The listing builds one solid part. Answer for the finished solid, in the listing's coordinates (mm). A direction names the side the tool comes from. Give positions to 0.01 mm unless a question says otherwise; leave off trailing zeros. Loops run counter-clockwise (first coordinate to the right, second up) from the corner with the lowest first, then second, coordinate; pieces in that order, holes last. Notation, with made-up numbers: M 9,74 L 25,74 A18 ccw 25,101 Z; hole C 73,78 d2. An arc over 180 degrees is marked long. Use one line per item in the form item = value. Start each with the question number.
1. The part is cut by section C-C (z = 10.75). Write down the section's boundary in (x, y), and give its area (3 significant figures).
2. The part is cut by section D-D (x = 7.25). Write down the section's boundary in (y, z), and give its area (3 significant figures).
3. Each of these flat-tipped pins is pushed along its axis until it touches: pin 1 Ø3 at (x, y) = (0, 12) entering from -Z; pin 2 Ø3 at (y, z) = (4, 0) entering from +X; pin 3 Ø2.5 at (y, z) = (14, 6.5) entering from +X. Where does it stop, or does it pass through?
4. Straight lines are drawn through the part: line 1 (Y direction, x = -3.75, z = 10); line 2 (Y direction, x = -4, z = 1); line 3 (Z direction, x = -5.25, y = 3). For each, find the intervals that lie inside material, in ascending order. Write a range as from..to.
5. The mould has two halves that part along Y. Classify faces 1 (the face through (5, 2.4, 4)), 2 (the face through (-3, 13, 9)), 3 (the face through (8, 9, 6)): released by +Y, released by -Y, zero draft, split by the parting line, or undercut.
6. The part is cut by section B-B (z = 0.5). Write down the section's boundary in (x, y).
7. The part is cut by section A-A (x = -5.5). Write down the section's boundary in (y, z).
8. For faces 4 (the face through (5, 5.75, 10)), 5 (the face through (-7.5, 12, 6)), 6 (the face through (-0.208, 13.586, 2.028)), 7 (the face through (-5, 2.4, 4)), 8 (the face through (0, 9, 9)), determine the directions among +Z, -Z, +X, -X, +Y, -Y from which every point of the face is accessible in a straight line to the end or side of a thin tool.
from build123d import *

# Parameters (mm, degrees)
BOSS_EXTRUDE1_DEPTH = 13
CUT_EXTRUDE1_DEPTH  = 9
SKETCH4_R           = 1.6
CUT_EXTRUDE2_DEPTH  = 20.448650339
SKETCH5_R           = 1.25
CUT_EXTRUDE3_DEPTH  = 22.592822882
CUT_EXTRUDE4_DEPTH  = 22.592822882
CUT_EXTRUDE5_DEPTH  = 7.8
SKETCH9_W           = 6.962435565
SKETCH9_H           = 4.2
CUT_EXTRUDE6_DEPTH  = 7.8
SKETCH10_R          = 1.4
BOSS_EXTRUDE2_DEPTH = 2.5
CHAMFER1_SIZE       = 0.5
BOSS_EXTRUDE3_START = 0.2
BOSS_EXTRUDE3_DEPTH = 0.2


with BuildPart() as part:
    # Sketch1 → Boss-Extrude1 (new body)
    with BuildSketch(Plane.XY):
        Polygon((-8.5, 0), (8.5, 0), (8.5, 9), (7.5, 9), (7.5, 15), (-7.5, 15), (-7.5, 9), (-8.5, 9), align=None)
    extrude(amount=BOSS_EXTRUDE1_DEPTH)

    # Sketch2 → Cut-Extrude1 (cut)
    with BuildSketch(Plane.XY.offset(13)):
        with BuildLine():
            Line((3, 18), (3, 12))
            ThreePointArc((3, 12), (0, 9), (-3, 12))
            Line((-3, 12), (-3, 18))
            ThreePointArc((-3, 18), (0, 21), (3, 18))
        make_face()
    extrude(amount=-CUT_EXTRUDE1_DEPTH, mode=Mode.SUBTRACT)

    # Sketch4 → Cut-Extrude2 (cut, through all)
    with BuildSketch(Plane.XY.offset(4)):
        with Locations((0, 12)):
            Circle(SKETCH4_R)
    extrude(amount=-CUT_EXTRUDE2_DEPTH, mode=Mode.SUBTRACT)

    # Sketch5 → Cut-Extrude3 (cut, through all)
    with BuildSketch(Plane.XY.offset(13)):
        with Locations((-4.75, 4.5)):
            Circle(SKETCH5_R)
        with Locations((4.75, 4.5)):
            Circle(SKETCH5_R)
    extrude(amount=-CUT_EXTRUDE3_DEPTH, mode=Mode.SUBTRACT)

    # Sketch7 → Cut-Extrude4 (cut, through all)
    with BuildSketch(Plane.XY.offset(13)):
        with BuildLine():
            Line((-6.75, 5.75), (-2.75, 5.75))
            ThreePointArc((-2.75, 5.75), (-1.5, 4.5), (-2.75, 3.25))
            Line((-2.75, 3.25), (-6.75, 3.25))
            ThreePointArc((-6.75, 3.25), (-8, 4.5), (-6.75, 5.75))
        make_face()
        with BuildLine():
            Line((6.75, 3.25), (2.75, 3.25))
            ThreePointArc((2.75, 3.25), (1.5, 4.5), (2.75, 5.75))
            Line((2.75, 5.75), (6.75, 5.75))
            ThreePointArc((6.75, 5.75), (8, 4.5), (6.75, 3.25))
        make_face()
    extrude(amount=-CUT_EXTRUDE4_DEPTH, mode=Mode.SUBTRACT)

    # Sketch8 → Cut-Extrude5 (cut)
    with BuildSketch(Plane(origin=(0, 0, 0), x_dir=(-1, 0, 0), z_dir=(0, 0, -1))):
        Polygon((-1.537564435, 6.6), (-3.962435565, 6.6), (-5.174871131, 4.5), (-3.962435565, 2.4), (-1.537564435, 2.4), (-0.325128869, 4.5), align=None)
        Polygon((1.537564435, 6.6), (0.325128869, 4.5), (1.537564435, 2.4), (3.962435565, 2.4), (5.174871131, 4.5), (3.962435565, 6.6), align=None)
    extrude(amount=-CUT_EXTRUDE5_DEPTH, mode=Mode.SUBTRACT)

    # Sketch9 → Cut-Extrude6 (cut)
    with BuildSketch(Plane(origin=(0, 0, 7.8), x_dir=(-1, 0, 0), z_dir=(0, 0, -1))):
        with Locations((5.018782218, 4.5)):
            Rectangle(SKETCH9_W, SKETCH9_H)
        with Locations((-5.018782218, 4.5)):
            Rectangle(SKETCH9_W, SKETCH9_H)
    extrude(amount=CUT_EXTRUDE6_DEPTH, mode=Mode.SUBTRACT)

    # Sketch10 → Boss-Extrude2 (add)
    with BuildSketch(Plane(origin=(0, 0, 0), x_dir=(-1, 0, 0), z_dir=(0, 0, -1))):
        with Locations(Location((0, 8.263139721, 0), (0, 0, 180))):
            Circle(SKETCH10_R)
        with Locations(Location((0, 2.263139721, 0), (0, 0, 150))):
            Circle(SKETCH10_R)
    extrude(amount=BOSS_EXTRUDE2_DEPTH)

    # Chamfer1
    chamfer1_edges = [part.edges().sort_by_distance(p)[0] for p in [
        (-1.4, 8.263139721, -2.5),
        (-1.212435565, 1.563139721, -2.5),
    ]]
    chamfer(chamfer1_edges, length=CHAMFER1_SIZE)

    # Sketch11 → Boss-Extrude3 (add)
    with BuildSketch(Plane.XY.offset(4).offset(BOSS_EXTRUDE3_START)):
        with BuildLine():
            Line((3, 15), (-3, 15))
            Line((-3, 15), (-3, 12))
            ThreePointArc((-3, 12), (0, 9), (3, 12))
            Line((3, 12), (3, 15))
        make_face()
    extrude(amount=-BOSS_EXTRUDE3_DEPTH)


solid = part.part
Derived:
q1.outline = M -8.5,0 L 8.5,0 L 8.5,9 L 7.5,9 L 7.5,15 L 3,15 L 3,12 A3 cw -3,12 L -3,15 L -7.5,15 L -7.5,9 L -8.5,9 Z; hole M -6.75,3.25 L -2.75,3.25 A1.25 ccw -2.75,5.75 L -6.75,5.75 A1.25 ccw Z; hole M 2.75,3.25 L 6.75,3.25 A1.25 ccw 6.75,5.75 L 2.75,5.75 A1.25 ccw Z
q1.area = 181 mm2
q2.outline = M 0,0 L 2.4,0 L 2.4,7.8 L 3.35,7.8 L 3.35,13 L 0,13 Z; M 5.65,7.8 L 6.6,7.8 L 6.6,0 L 15,0 L 15,13 L 5.65,13 Z
q2.area = 150 mm2
q3.pin_1 = 4
q3.pin_2 = 1.48
q3.pin_3 = 7.5
q4.line_1 = 0..3.25, 5.75..15
q4.line_2 = 0..2.4, 6.6..15
q4.line_3 = 7.8..13
q5.face_1 = undercut
q5.face_2 = zero draft
q5.face_3 = released by +Y
q6.outline = M -8.5,0 L 8.5,0 L 8.5,2.4 L 1.54,2.4 L 0.33,4.5 L 1.54,6.6 L 8.5,6.6 L 8.5,9 L 7.5,9 L 7.5,15 L -7.5,15 L -7.5,9 L -8.5,9 L -8.5,6.6 L -1.54,6.6 L -0.33,4.5 L -1.54,2.4 L -8.5,2.4 Z; hole C 0,12 d3.2
q7.outline = M 0,0 L 2.4,0 L 2.4,7.8 L 3.25,7.8 L 3.25,13 L 0,13 Z; M 5.75,7.8 L 6.6,7.8 L 6.6,0 L 15,0 L 15,13 L 5.75,13 Z
q8.face_4 = +Z, -Z
q8.face_5 = +Z, -Z, -X, +Y
q8.face_6 = -Z
q8.face_7 = -Z, -X
q8.face_8 = +Z, +Y
